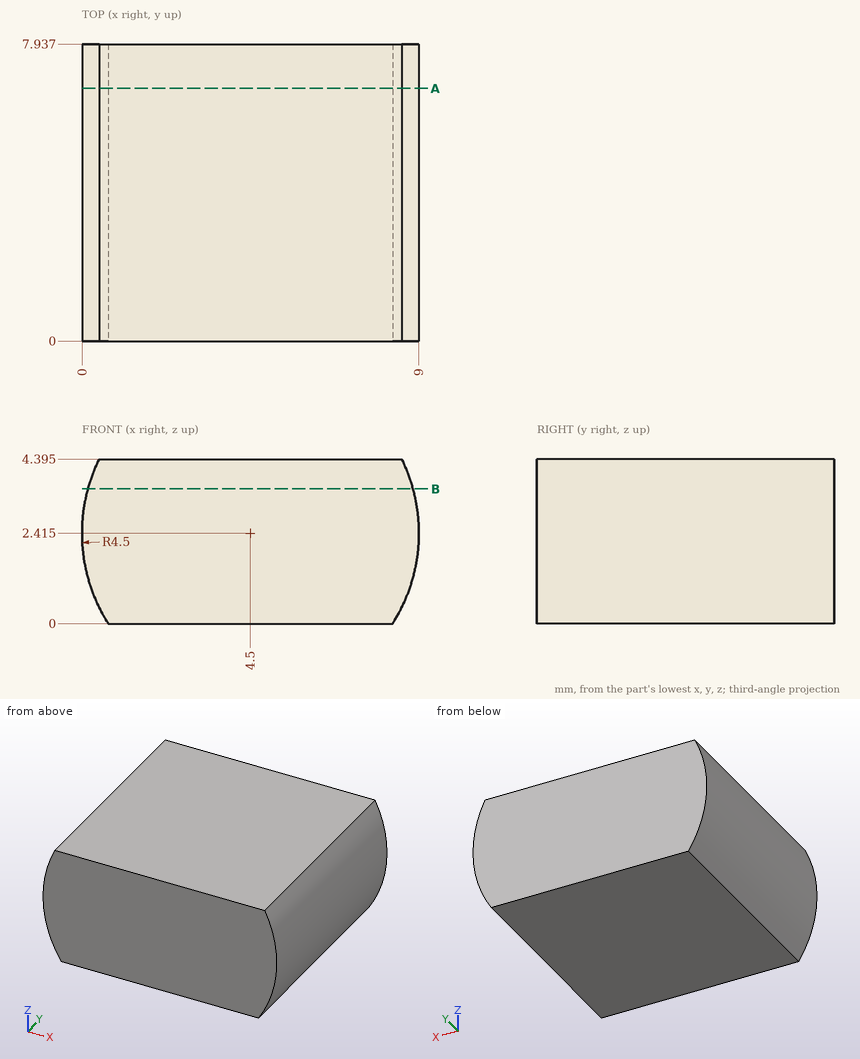
Answer from the drawing. Dimensions are ordinates in mm from the lowest x, y and z of the part. Coordinates: 2 decimals unless noted, no trailing zeros. Order: outer loops, then holes, each group sorted by start corner. A loop starts at its lowest first (then second) coordinate and runs counter-clockwise, first axis right, second up. Notation, with made-up numbers: (74, 20.25) - (108, 20.25) arc R18 cw to (108, 49.25) - close; hole circle Ø1 at (-21.5, -33.5). An arc over 180 degrees is marked (long way). Put each result on its own line as item: value. Start each with the question number.
1) Find section B-B (z = 3.6). Give the vertices of the cut face in (x, y), plus the area to 3 significant figures.
2) Find section A-A (y = 6.75). Give the vertices of the cut face in (x, z) (1 decimal), plus the area to 3 significant figures.
3) Find the intervals of material crossed by line 1 (X direction, y = 4.5, z = 2.2) (1 decimal); line 2 (X direction, y = 2.5, z = 3.6), in increasing order. Write a range as from..to.
Results list:
1. outline: (0.16, 0) - (8.84, 0) - (8.84, 7.94) - (0.16, 7.94) - close
1. area: 68.9 mm^2
2. outline: (0.5, 4.4) arc R4.5 ccw to (0.7, 0) - (8.3, 0) arc R4.5 ccw to (8.5, 4.4) - close
2. area: 37.9 mm^2
3. line 1: x = 0..9
3. line 2: x = 0.16..8.84
